```python
from build123d import *

# Parameters (mm, degrees)
F1_DEPTH = 5


with BuildPart() as f1:
    # F0 (on Top) → F1 (new body)
    with BuildSketch(Plane.XY):
        with BuildLine():
            ThreePointArc((-25, 0), (-18.873774, 1.868872), (-12.5, 2.5))
            Line((-12.5, 2.5), (-12.5, 11))
            Line((-12.5, 11), (-29.5, 11))
            Line((-29.5, 11), (-25, 0))
        make_face()
        with BuildLine():
            ThreePointArc((-12.5, 2.5), (-6.126226, 1.868872), (0, 0))
            Line((0, 0), (4.5, 11))
            ThreePointArc((4.5, 11), (-12.5, 18), (-29.5, 11))
            Line((-29.5, 11), (-12.5, 11))
            Line((-12.5, 11), (-12.5, 2.5))
        make_face()
    extrude(amount=F1_DEPTH)


solid = f1.part
```
Verification items for the finished model (mm, model axes). Coordinates: 2 decimals unless noted, no trailing zeros. Order: outer loops, then holes, each group sorted by start corner. A loop starts at its lowest first (then second) coordinate and runs counter-clockwise, first axis right, second up. Notation, with made-up numbers: (77, 87) -> (126, 87) arc R23 ccw to (126, 110) -> close; hole circle Ø6 at (-0.75, 52). An arc over 180 degrees is marked (long way). Put each result on its own line as item: value. Start each with the question number.
1) Material ranges on L1, parallel to Y at x = -12, z = 3.7; L2, parallel to X at y = 7, z = 0.8; L3, parallel to X at y = 4.25, z = 0.85, recorded low to high.
2) Cross-section at A-A (y = 1). Enter the section's corners in (x, z).
3) Go/stop test with flat-tipped pins: pin 1 (1 mm diameter, centred on x = -9.5, z = 2, fed in from +Y); pin 2 (1.5 mm diameter, centred on y = 7.5, z = 3.5, fed in from +X) (3 decimals); pin 3 (3 mm diameter, centred on y = 13, z = 1.5, fed in from +X). Record where each tip stops, or that it passes through.
4) Cross-section at B-B (z = 2.25). Enter the section's corners in (x, y).
5) Cross-section at D-D (y = 5.75). Enter the section's corners in (x, z).
6) Cross-section at C-C (x = -9). Enter the section's corners in (y, z), plus the area to 3 significant figures.
Geometry check:
1. L1: y = 2.5 to 17.99
1. L2: x = -27.86 to 2.86
1. L3: x = -26.74 to 1.74
2. outline: (-25.41, 0) -> (-22.26, 0) -> (-22.26, 5) -> (-25.41, 5) -> close; (-2.74, 0) -> (0.41, 0) -> (0.41, 5) -> (-2.74, 5) -> close
3. pin 1: stops at y = 17.87
3. pin 2: stops at x = 3.375
3. pin 3: stops at x = 3.98
4. outline: (-29.5, 11) -> (-25, 0) arc R32.5 cw to (0, 0) -> (4.5, 11) arc R24.14 ccw to start
5. outline: (-27.35, 0) -> (2.35, 0) -> (2.35, 5) -> (-27.35, 5) -> close
6. outline: (2.31, 0) -> (17.74, 0) -> (17.74, 5) -> (2.31, 5) -> close
6. area: 77.2 mm^2
